Verification items for the finished model (mm, model axes). A direction names the side the tool comes from. Give positions to 0.01 mm unless a question says otherwise; leave off trailing zeros. Order: outer loops, then holes, each group sorted by start corner. A loop starts at its lowest first (then second) coordinate and runs counter-clockwise, first axis right, second up. Notation, with made-up numbers: M -24.75,77 L -1.75,77 A17 cw -1.75,103 Z; hole C 52,63 d2. An arc over 180 degrees is marked long. Answer as a JSON object with one key per item and string values.
```python
from build123d import *

# Parameters (mm, degrees)
SKETCH_1_R          = 2.4999999999999982
SKETCH_1_R_2        = 2.5000000000000027
EXTRUDE_1_DEPTH     = 5.1
SKETCH_2_R          = 4.999999999999998
SKETCH_2_R_2        = 2.5
EXTRUDE_2_DEPTH     = 5.94
CUT_EXTRUDE_1_DEPTH = 3.5
CUT_EXTRUDE_START   = -0.6
CUT_EXTRUDE_3_DEPTH = 0.6
EXTRUDE_START       = 1.2
SKETCH_6_R          = 4.999999999999998
SKETCH_6_R_2        = 2.5
SKETCH_6_R_3        = 5
SKETCH_6_R_4        = 2.4999999999999987
EXTRUDE_4_DEPTH     = 1.2
SKETCH_7_R          = 2.6000000000000005
CUT_EXTRUDE_4_DEPTH = 33.57721194023454
SKETCH_8_R          = 2.6
CUT_EXTRUDE_5_DEPTH = 31.8406734329677


with BuildPart() as part:
    # Эскиз1 → Бобышка-Вытянуть1 (new body)
    with BuildSketch(Plane(origin=(0, 0, 0), x_dir=(1, 0, 0), z_dir=(0, 1, 0))):
        with BuildLine():
            Line((6.718023264525762, 8.928267668376021), (7.161238337218641, 11.37785065819786))
            Line((7.161238337218641, 11.37785065819786), (7.294846288705666, 12.560700282216452))
            Line((7.294846288705666, 12.560700282216452), (7.085001061393901, 12.665407082864023))
            Line((7.085001061393901, 12.665407082864023), (6.15987792536569, 11.916319971156167))
            Line((6.15987792536569, 11.916319971156167), (5.853623131200735, 12.10383694173367))
            Line((5.853623131200735, 12.10383694173367), (5.855060736117009, 13.29420757772634))
            Line((5.855060736117009, 13.29420757772634), (5.634886528714601, 13.37496556136943))
            Line((5.634886528714601, 13.37496556136943), (4.798663389284832, 12.527784837542624))
            Line((4.798663389284832, 12.527784837542624), (4.473480547373511, 12.680135526842204))
            Line((4.473480547373511, 12.680135526842204), (4.342730025112913, 13.863304415323501))
            Line((4.342730025112913, 13.863304415323501), (4.114949999467502, 13.919114749889351))
            Line((4.114949999467502, 13.919114749889351), (3.3779694438823102, 12.984318526945106))
            Line((3.3779694438823102, 12.984318526945106), (3.0378804853992434, 13.099618628946285))
            Line((3.0378804853992434, 13.099618628946285), (2.776558986480811, 14.260952083189514))
            Line((2.776558986480811, 14.260952083189514), (2.54399037483231, 14.291124494483034))
            Line((2.54399037483231, 14.291124494483034), (1.9153675367628848, 13.280274532718662))
            Line((1.9153675367628848, 13.280274532718662), (1.56457875493138, 13.35709799101592))
            Line((1.56457875493138, 13.35709799101592), (1.175918359734634, 14.482232389631033))
            Line((1.175918359734634, 14.482232389631033), (0.9414376205823001, 14.486393698794194))
            Line((0.9414376205823001, 14.486393698794194), (0.4289474421954887, 13.411992407470256))
            Line((0.42894744219548875, 13.411992407470256), (0.07179746795026506, 13.449389053044667))
            Line((0.07179746795026506, 13.449389053044667), (-0.4393947883485354, 14.524408492330128))
            Line((-0.43939478834853546, 14.524408492330128), (-0.6728875469021285, 14.502507231398162))
            Line((-0.6728875469021285, 14.502507231398162), (-1.062906477097084, 13.377843036257644))
            Line((-1.062906477097084, 13.377843036257644), (-1.4220003362283888, 13.375350339371238))
            Line((-1.4220003362283888, 13.375350339371238), (-2.049401918098927, 14.386958748197415))
            Line((-2.049401918098927, 14.386958748197415), (-2.279018807507275, 14.33926579666565))
            Line((-2.279018807507275, 14.33926579666565), (-2.5417426516817105, 13.178248785832608))
            Line((-2.5417426516817105, 13.178248785832608), (-2.898339045786024, 13.13589757669542))
            Line((-2.898339045786024, 13.13589757669542), (-3.6341901158202092, 14.071583165165732))
            Line((-3.6341901158202092, 14.071583165165732), (-3.8570911851181764, 13.998688399693854))
            Line((-3.8570911851181764, 13.998688399693854), (-3.989270518385492, 12.815678280718325))
            Line((-3.989270518385492, 12.815678280718325), (-4.3389589867331635, 12.733992368173748))
            Line((-4.3389589867331635, 12.733992368173748), (-5.174158380979493, 13.582182376127184))
            Line((-5.174158380979493, 13.582182376127184), (-5.3875867419063175, 13.48498737481814))
            Line((-5.3875867419063175, 13.48498737481814), (-5.3875867419063175, 12.2946158707315))
            Line((-5.3875867419063175, 12.2946158707315), (-5.751610974482103, 12.12883970299033))
            Line((-5.751610974482103, 12.12883970299033), (-6.666748566138722, 12.905854249247858))
            Line((-6.666748566138722, 12.905854249247858), (-7.13096440438616, 12.63943472468846))
            Line((-7.13096440438616, 12.63943472468846), (-7.025830916712447, 12.175864106991055))
            ThreePointArc((-7.025830916712449, 12.175864106991055), (-10.264322646127633, 9.799709596012173), (-12.51111253150909, 6.470163958468902))
            Line((-12.51111253150909, 6.470163958468902), (-5.241071220187256, 3.924995297345621))
            Line((-5.241071220187256, 3.924995297345621), (-4.737733567637334, 1.5980865565051285))
            ThreePointArc((-4.737733567637334, 1.5980865565051288), (-4.061430338102922, -2.9162962141622684), (1.55e-15, -5))
            Line((2.2e-16, -5), (21.46693589645179, -5.388260461869603))
            ThreePointArc((21.46693589645179, -5.388260461869605), (26.46693589645179, -0.3882604618696045), (21.46693589645179, 4.611739538130397))
            Line((21.46693589645179, 4.611739538130397), (7.924308406385933, 7.062073595968816))
            ThreePointArc((7.924308406385932, 7.062073595968816), (7.00463576208043, 7.790569444059032), (6.718023264525762, 8.928267668376021))
        make_face()
        with Locations(Location((21.46693589645179, -0.38826046186960367, 0), (0, 0, 270))):
            Circle(SKETCH_1_R, mode=Mode.SUBTRACT)
        with Locations(Location((-2.78e-15, -1.44e-15, 0), (0, 0, 270))):
            Circle(SKETCH_1_R_2, mode=Mode.SUBTRACT)
    extrude(amount=EXTRUDE_1_DEPTH)

    # Эскиз2 → Бобышка-Вытянуть2 (add)
    with BuildSketch(Plane(origin=(0, 5.1, 0), x_dir=(1, 0, 0), z_dir=(0, 1, 0))):
        with Locations(Location((0, 0, 0), (0, 0, 270))):
            Circle(SKETCH_2_R)
        with Locations(Location((0, 0, 0), (0, 0, 270))):
            Circle(SKETCH_2_R_2, mode=Mode.SUBTRACT)
    extrude(amount=EXTRUDE_2_DEPTH)

    # Эскиз4 → Вырез-Вытянуть1 (cut)
    with BuildSketch(Plane.XZ):
        with BuildLine():
            Line((-5.241071220187255, -3.924995297345621), (-7.025830916712447, -12.175864106991055))
            ThreePointArc((-7.025830916712447, -12.175864106991055), (-10.264322646127628, -9.799709596012166), (-12.511112531509088, -6.470163958468901))
            Line((-12.511112531509088, -6.470163958468901), (-5.241071220187255, -3.924995297345621))
        make_face()
    extrude(amount=-CUT_EXTRUDE_1_DEPTH, mode=Mode.SUBTRACT)

    # Эскиз5 → Вырез-Вытянуть3 (cut)
    with BuildSketch(Plane(origin=(0, 5.1, 0), x_dir=(1, 0, 0), z_dir=(0, 1, 0)).offset(CUT_EXTRUDE_START)):
        with BuildLine():
            Line((-5.241071220187255, 3.924995297345621), (-7.025830916712447, 12.175864106991055))
            ThreePointArc((-7.025830916712447, 12.175864106991055), (-10.264322646127628, 9.799709596012168), (-12.511112531509088, 6.470163958468901))
            Line((-12.511112531509088, 6.470163958468901), (-5.241071220187255, 3.924995297345621))
        make_face()
    extrude(amount=CUT_EXTRUDE_3_DEPTH, mode=Mode.SUBTRACT)

    # Эскиз6 → Бобышка-Вытянуть4 (add)
    # profile 1 of 2: a face of its own
    with BuildSketch(Plane.XZ.offset(EXTRUDE_START)):
        with Locations(Location((0, 0, 0), (0, 0, 270))):
            Circle(SKETCH_6_R)
        with Locations(Location((0, 0, 0), (0, 0, 270))):
            Circle(SKETCH_6_R_2, mode=Mode.SUBTRACT)
    # profile 2 of 2: a face of its own
    with BuildSketch(Plane.XZ.offset(EXTRUDE_START)):
        with Locations(Location((21.46693589645179, 0.38826046186960295, 0), (0, 0, 270))):
            Circle(SKETCH_6_R_3)
        with Locations(Location((21.46693589645179, 0.38826046186960295, 0), (0, 0, 270))):
            Circle(SKETCH_6_R_4, mode=Mode.SUBTRACT)
    extrude(amount=-EXTRUDE_4_DEPTH)

    # Эскиз7 → Вырез-Вытянуть4 (cut, through all)
    with BuildSketch(Plane(origin=(0, 11.04, 0), x_dir=(1, 0, 0), z_dir=(0, 1, 0))):
        with Locations(Location((0, 0, 0), (0, 0, 270))):
            Circle(SKETCH_7_R)
    extrude(amount=-CUT_EXTRUDE_4_DEPTH, mode=Mode.SUBTRACT)

    # Эскиз8 → Вырез-Вытянуть5 (cut, through all)
    with BuildSketch(Plane(origin=(0, 5.1, 0), x_dir=(1, 0, 0), z_dir=(0, 1, 0))):
        with Locations(Location((21.46693589645179, -0.38826046186960295, 0), (0, 0, 270))):
            Circle(SKETCH_8_R)
    extrude(amount=-CUT_EXTRUDE_5_DEPTH, mode=Mode.SUBTRACT)


solid = part.part
```
Q1. Tool access check on faces 5 (the face through (14.79, 2.51, -5.82)), 6 (the face through (6.937, 2.514, -10.136)), 7 (the face through (-3.92, 2.51, -13.42)). Record the directions out of +Z, -Z, +X, -X, +Y, -Y that give a thin tool (end or side, any length) a straight path to the whole face; none if there is none.
Resolved:
{"face 5": "-Z, +X, +Y, -Y", "face 6": "+X, +Y, -Y", "face 7": "-Z, +Y, -Y"}
Q2. Section check D-D on z = -5.5. Record the cut outline in (x, y), then the cut area to 3 significant figures.
Resolved:
{"outline": "M -9.74,3.5 L -5.58,3.5 L -5.58,0 L 16.56,0 L 16.56,5.1 L -5.58,5.1 L -5.58,4.5 L -9.74,4.5 Z", "area": "117 mm²"}
Q3. Release check for a two-part mould opening along X. For faces 1 (the face through (-8.927, 3.993, -5.215)), 2 (the face through (-2, 11.04, 2)), 3 (the face through (4.41, 2.51, -13.26)), 4 (the face through (1.373, 2.514, -13.912)) record: +X half, -X half, draft (parallel to the pull), parting line (faces both ways), or undercut.
Resolved:
{"face 1": "-X half", "face 2": "draft", "face 3": "undercut", "face 4": "undercut"}
Q4. Section check C-C on y = 6.25. Record the cut outline in (x, z), then the cut area to 3 significant figures.
Resolved:
{"outline": "C 0,0 d10; hole C 0,0 d5.2", "area": "57.3 mm²"}
Q5. Gauge pin test, flat ends, axial feed: pin 1 Ø2 at (x, z) = (-9, -7.5) entering from -Y; pin 2 Ø1.5 at (x, y) = (-7.5, 4) entering from +Z; pin 3 Ø1.5 at (x, y) = (0.5, 9.5) entering from -Z. Record the tip position at first contact, or that the pin passes through.
Resolved:
{"pin 1": "stops at y = 3.5", "pin 2": "stops at z = -4.45", "pin 3": "stops at z = -5"}
Q6. Section check A-A on x = 22.5. Record the cut outline in (y, z), then the cut area to 3 significant figures.
Resolved:
{"outline": "M -1.2,-4.5 L 5.1,-4.5 L 5.1,-2 L -1.2,-2 Z; M -1.2,2.77 L 5.1,2.77 L 5.1,5.28 L -1.2,5.28 Z", "area": "31.6 mm²"}
Q7. Material ranges on L1, parallel to X at y = 5.5, z = 0; L2, parallel to X at y = 2.5, z = 1; L3, parallel to X at y = 7.25, z = -2.25, recorded low to high.
Resolved:
{"L1": "x = -5 to -2.6, 2.6 to 5", "L2": "x = -4.9 to -2.4, 2.4 to 18.94, 23.99 to 26.43", "L3": "x = -4.47 to -1.3, 1.3 to 4.47"}
